Geometry check sheet. Reference: the model listing, model coordinates, mm. A direction names the side the tool comes from. Give positions to 0.01 mm unless a question says otherwise; leave off trailing zeros. Loops run counter-clockwise (first coordinate to the right, second up) from the corner with the lowest first, then second, coordinate; pieces in that order, holes last. Notation, with made-up numbers: (51, -20) -> (91, -20) arc R26 cw to (91, -3) -> close; hole circle Ø3 at (-11, 32.5). An arc over 180 degrees is marked (long way). Write each question's results on one line, items separated by ' | '. Start each with the question number.
1) Draft check along Z on faces 3 (the face through (0, 15, 3.8)), 4 (the face through (-24, 15, 0)), 5 (the face through (-0.15, 15.21, -15.5)). Enter one of: pulls with the +Z half, pulls with the -Z half, needs draft (parallel to the pull), parting line crosses it, or undercut.
2) Sectioned sample at A-A on x = 17. Record the cut outline in (y, z), then the cut area to 3 significant figures.
3) Sectioned sample at C-C on z = 11. Record the cut outline in (x, y), then the cut area to 3 significant figures.
4) Depth check by flat-ended pin: pin 1 (9.5 mm diameter, centred on x = 17, y = 15, fed in from -Z). Enter the tip coordinate at first touch or a pass-through.
5) Set-up check for faces 1 (the face through (0, 30, 0)), 2 (the face through (0, 15, 14.2)): record each of +Z, -Z, +X, -X, +Y, -Y from which the full face is reachable in a straight line by a thin tool's end or side.
6) Sectioned sample at B-B on y = 7.5. Record the cut outline in (x, z), then the cut area to 3 significant figures.
7) Scan lines: line 1 (Y direction, x = -17, z = -14.5); line 2 (Z direction, x = -18, y = 6.5); line 3 (Z direction, x = 0, y = 22.25). Record each from-to range of solid material in increasing order. Write a range as from..to.
8) Sectioned sample at D-D on y = 15. Record the cut outline in (x, z), then the cut area to 3 significant figures.
```python
from build123d import *

# Parameters (mm, degrees)
SKETCH1_W               = 48
SKETCH1_H               = 45
BOSS_EXTRUDE1_DEPTH     = 30
SKETCH2_W               = 10.4
SKETCH2_H               = 20.4
CUT_EXTRUDE1_DEPTH      = 49
SKETCH3_R               = 4.15
CUT_EXTRUDE2_DEPTH      = 46
CUT_EXTRUDE3_DEPTH      = 1
CUT_EXTRUDE3_DEPTH_BACK = 31


with BuildPart() as part:
    # Sketch1 → Boss-Extrude1 (new body)
    with BuildSketch(Plane(origin=(0, 0, 0), x_dir=(1, 0, 0), z_dir=(0, 1, 0))):
        Rectangle(SKETCH1_W, SKETCH1_H)
    extrude(amount=BOSS_EXTRUDE1_DEPTH)

    # Sketch2 → Cut-Extrude1 (cut, through all)
    with BuildSketch(Plane(origin=(24, 0, 0), x_dir=(0, 0, -1), z_dir=(1, 0, 0))):
        with Locations((-9, 15)):
            Rectangle(SKETCH2_W, SKETCH2_H)
    extrude(amount=-CUT_EXTRUDE1_DEPTH, mode=Mode.SUBTRACT)

    # Sketch3 → Cut-Extrude2 (cut, through all)
    with BuildSketch(Plane.XY.offset(22.5)):
        with Locations((-17, 15)):
            Circle(SKETCH3_R)
        with Locations((17, 15)):
            Circle(SKETCH3_R)
    extrude(amount=-CUT_EXTRUDE2_DEPTH, mode=Mode.SUBTRACT)

    # Sketch4 → Cut-Extrude3 (cut, two sides)
    with BuildSketch(Plane(origin=(0, 30, 0), x_dir=(1, 0, 0), z_dir=(0, 1, 0))) as cut_extrude3_sk:
        with BuildLine():
            Line((-7, 141.788608739), (-7, 22.5))
            ThreePointArc((-7, 22.5), (0, 15.5), (7, 22.5))
            Line((7, 22.5), (7, 141.788608739))
            Line((7, 141.788608739), (7, 380.365826216))
            Line((7, 380.365826216), (-7, 380.365826216))
            Line((-7, 380.365826216), (-7, 141.788608739))
        make_face()
    extrude(amount=CUT_EXTRUDE3_DEPTH, mode=Mode.SUBTRACT)
    extrude(cut_extrude3_sk.sketch, amount=-CUT_EXTRUDE3_DEPTH_BACK, mode=Mode.SUBTRACT)


solid = part.part
```
Result:
1) face 3: undercut | face 4: needs draft | face 5: pulls with the -Z half
2) outline: (0, -22.5) -> (10.85, -22.5) -> (10.85, 3.8) -> (4.8, 3.8) -> (4.8, 14.2) -> (10.85, 14.2) -> (10.85, 22.5) -> (0, 22.5) -> close; (19.15, -22.5) -> (30, -22.5) -> (30, 22.5) -> (19.15, 22.5) -> (19.15, 14.2) -> (25.2, 14.2) -> (25.2, 3.8) -> (19.15, 3.8) -> close | area: 851 mm^2
3) outline: (-24, 0) -> (24, 0) -> (24, 4.8) -> (-24, 4.8) -> close; (-24, 25.2) -> (24, 25.2) -> (24, 30) -> (-24, 30) -> close | area: 461 mm^2
4) pin 1: z = -22.5
5) face 1: +Z, -Z, +X, -X, +Y | face 2: +X, -X
6) outline: (-24, -22.5) -> (-7, -22.5) arc R7 cw to (7, -22.5) -> (24, -22.5) -> (24, 3.8) -> (-24, 3.8) -> close; (-24, 14.2) -> (24, 14.2) -> (24, 22.5) -> (-24, 22.5) -> close | area: 1,580 mm^2
7) line 1: 0..10.85, 19.15..30 | line 2: -22.5..3.8, 14.2..22.5 | line 3: -15.5..3.8, 14.2..22.5
8) outline: (-24, -22.5) -> (-21.15, -22.5) -> (-21.15, 3.8) -> (-24, 3.8) -> close; (-24, 14.2) -> (-21.15, 14.2) -> (-21.15, 22.5) -> (-24, 22.5) -> close; (-12.85, -22.5) -> (-7, -22.5) arc R7 cw to (7, -22.5) -> (12.85, -22.5) -> (12.85, 3.8) -> (-12.85, 3.8) -> close; (-12.85, 14.2) -> (12.85, 14.2) -> (12.85, 22.5) -> (-12.85, 22.5) -> close; (21.15, -22.5) -> (24, -22.5) -> (24, 3.8) -> (21.15, 3.8) -> close; (21.15, 14.2) -> (24, 14.2) -> (24, 22.5) -> (21.15, 22.5) -> close | area: 1,010 mm^2
